The model under review builds one solid part; all positions refer to its coordinate system, in mm. Give positions to 0.01 mm unless a question says otherwise; leave off trailing zeros. Write each loop counter-clockwise with the first axis right and the second up, starting at its lowest first coordinate (ties: lowest second). Pieces come first, ordered by that corner, then holes. Notation, with made-up numbers: (-12.5, 45) -> (1.5, 45) arc R15 cw to (1.5, 52) -> close; hole circle Ø2 at (43, 84). An arc over 180 degrees is marked (long way). Use CSV: the item, a comma, the result in double quotes.
Autodesk Inventor part; units mm, degrees
ref_plane "YZ Plane" through (0, 0, 0) normal (1, 0, 0) x (0, 1, 0)
ref_plane "XZ Plane" through (0, 0, 0) normal (0, 1, 0) x (-1, 0, 0)
ref_plane "XY Plane" through (0, 0, 0) normal (0, 0, 1) x (1, 0, 0)
sketch "Sketch1" plane through (0, 0, 0) normal (0, 1, 0) x (-1, 0, 0)
  line L0 (-30, -30) -> (30, -30)
  line L1 (30, -30) -> (30, 30)
  line L2 (30, 30) -> (-30, 30)
  line L3 (-30, 30) -> (-30, -30)
  line L4 (-30, -30) -> (30, 30) construction
  line L5 (30, -30) -> (-30, 30) construction
  circle A0 centre (0, 0) radius 7.5
  dimension "d0" = 60
  dimension "d1" = 60
  dimension "d13" = 15
extrude "Extrusion1" add sketch "Sketch1" along normal blind 8
sketch "Sketch2" plane through (0, 8, 0) normal (0, 1, 0) x (1, 0, 0)
  line L0 (30, 30) -> (-30, 30)
  line L1 (-30, 30) -> (-30, -30)
  line L2 (-30, -30) -> (30, -30)
  line L3 (30, -30) -> (30, 30)
  line L4 (17.5, -17.5) -> (-17.5, -17.5)
  line L5 (-17.5, -17.5) -> (-17.5, 17.5)
  line L6 (-17.5, 17.5) -> (17.5, 17.5)
  line L7 (17.5, 17.5) -> (17.5, -17.5)
  line L8 (17.5, -17.5) -> (-17.5, 17.5) construction
  line L9 (-17.5, -17.5) -> (17.5, 17.5) construction
  line L10 (0, -17.5) -> (0, 17.5)
  line L11 (-17.5, 0) -> (17.5, 0)
  point P0 (0, 0)
  dimension "d4" = 35
  dimension "d5" = 35
hole "Hole1" at (-17.5, 8, 17.5) at (-17.5, 8, -17.5) at (17.5, 8, -17.5) at (17.5, 8, 17.5) direction (0, -1, 0) diameter 3.9 depth 10 tip angle 118
chamfer "Chamfer1" distance 2 angle 45 4 edges at (30, 4, 30) (30, 4, -30) (-30, 4, -30) (-30, 4, 30)
sketch "Sketch3" plane through (0, 8, 0) normal (0, 1, 0) x (1, 0, 0)
  line L0 (-28, -30) -> (-30, -28)
  line L1 (-28, -30) -> (28, -30)
  line L2 (30, -28) -> (28, -30)
  line L3 (30, -28) -> (30, 28)
  line L4 (28, 30) -> (30, 28)
  line L5 (28, 30) -> (-28, 30)
  line L6 (-30, 28) -> (-28, 30)
  line L7 (-30, 28) -> (-30, -28)
  circle A0 centre (17.5, 17.5) radius 1.95
  circle A1 centre (-17.5, -17.5) radius 1.95
  circle A2 centre (-17.5, 17.5) radius 1.95
  circle A3 centre (17.5, -17.5) radius 1.95
  circle A4 centre (0, 0) radius 7.5
  line L8 (25, -25) -> (-25, -25)
  line L9 (-25, -25) -> (-25, 25)
  line L10 (-25, 25) -> (25, 25)
  line L11 (25, 25) -> (25, -25)
  line L12 (25, -25) -> (-25, 25) construction
  line L13 (-25, -25) -> (25, 25) construction
  dimension "d17" = 50
  dimension "d18" = 50
hole "Hole2" at (-25, 8, -25) at (25, 8, -25) at (25, 8, 25) at (-25, 8, 25) direction (0, -1, 0) diameter 4.65 end through all
sketch "Sketch4" plane through (30, 0, 28) normal (1, 0, 0) x (0, 0, -1)
  line L0 (56, 8) -> (56, 0)
  line L1 (0, 8) -> (56, 8)
  line L2 (0, 0) -> (0, 8)
  line L3 (0, 0) -> (56, 0)
  circle A0 centre (28, 4) radius 1.5
  line L4 (-2, 8) -> (-2, 0)
  point P0 (28, 0)
  dimension "d26" = 3
  dimension "d27" = 4
  dimension "d28" = 30
extrude "Extrusion2" cut sketch "Sketch4" against normal through all contours A0
properties part number "00_XY_stage-CHUO_SEIKI_LD-647-R1-Top"
Q1. Consider section D-D (x = -1.5). Write out the cut boundary in (y, z).
Derived:
outline,"(0, -30) -> (8, -30) -> (8, -7.35) -> (0, -7.35) -> close; (0, 7.35) -> (8, 7.35) -> (8, 30) -> (0, 30) -> close"
Q2. Consider section C-C (z = 0). Write out the cut boundary in (x, y).
Derived:
outline,"(-30, 0) -> (-7.5, 0) -> (-7.5, 2.5) -> (-30, 2.5) -> close; (-30, 5.5) -> (-7.5, 5.5) -> (-7.5, 8) -> (-30, 8) -> close; (7.5, 0) -> (30, 0) -> (30, 2.5) -> (7.5, 2.5) -> close; (7.5, 5.5) -> (30, 5.5) -> (30, 8) -> (7.5, 8) -> close"
Q3. Consider section B-B (y = 4). State how many separate pieces and enclosed holes the cut face has, then the cut area to 3 significant figures.
Derived:
separate pieces,"2"
enclosed holes,"8"
area,"3,160 mm2"
Q4. The part is to be moulded in two halves that separate along X. For faces 1 (the cylindrical face through (-6.93, 3.94, 2.87)), 2 (the flat face through (0, 4, 30)), 3 (the flat face through (-29, 4, 29)), say which applies: pulls with the +X half, pulls with the -X half, needs draft (parallel to the pull), parting line crosses it, or undercut.
Derived:
face 1,"undercut"
face 2,"needs draft"
face 3,"pulls with the -X half"
Q5. Consider section A-A (x = -25). Write out the cut boundary in (y, z) (3 decimals).
Derived:
outline,"(0, -30) -> (8, -30) -> (8, -27.325) -> (0, -27.325) -> close; (0, -22.675) -> (8, -22.675) -> (8, 22.675) -> (0, 22.675) -> close; (0, 27.325) -> (8, 27.325) -> (8, 30) -> (0, 30) -> close; hole circle Ø3 at (4, 0)"
Q6. Insertion check: pin 1 (5 mm diameter, centred on x = 17.5, z = -17.5, fed in from +Y); pin 2 (3.5 mm diameter, centred on x = -25, z = 25, fed in from -Y). Each pin has a flat end and moves straight along its axis. Give the tip position at first contact, or say it passes through.
Derived:
pin 1,"stops at y = 8"
pin 2,"passes through"
Q7. To check wall thickness, follow probe 1 along X at (y, z) = (3.5, -25) (3 decimals); probe 2 along X at (y, z) = (4.5, -17.5); probe 3 along Y at (x, z) = (15.25, 0). State the ranges of each line that lie inside material, in increasing order.
Derived:
probe 1,"x = -30 to -27.325, -22.675 to 22.675, 27.325 to 30"
probe 2,"x = -30 to -19.45, -15.55 to 15.55, 19.45 to 30"
probe 3,"y = 0 to 2.5, 5.5 to 8"
